```python
from build123d import *

# Parameters (mm, degrees)
SKETCH_2_W          = 66
SKETCH_2_H          = 32
EXTRUDE_1_DEPTH     = 5
SKETCH_3_W          = 46
SKETCH_3_H          = 11.5
CUT_EXTRUDE_2_DEPTH = 38.013511047
SKETCH_4_W          = 5
SKETCH_4_H          = 11.5
CUT_EXTRUDE_3_DEPTH = 69.095521145
SKETCH_5_W          = 10
SKETCH_5_H          = 32
EXTRUDE_2_DEPTH     = 5
SKETCH_6_W          = 10
SKETCH_6_H          = 32
EXTRUDE_3_DEPTH     = 3
SKETCH_7_R          = 1.5
CUT_EXTRUDE_4_DEPTH = 39.013155617
CHAMFER_1_SIZE      = 2
CHAMFER_2_SIZE      = 1


with BuildPart() as part:
    # Sketch 2 → Extrude 1 (new body)
    with BuildSketch(Plane(origin=(0, 0, 0), x_dir=(0, 0, -1), z_dir=(1, 0, 0))):
        Rectangle(SKETCH_2_W, SKETCH_2_H)
    extrude(amount=EXTRUDE_1_DEPTH)

    # Sketch 3 → Cut-Extrude 2 (cut, through all)
    with BuildSketch(Plane.ZY):
        Rectangle(SKETCH_3_W, SKETCH_3_H)
    extrude(amount=-CUT_EXTRUDE_2_DEPTH, mode=Mode.SUBTRACT)

    # Sketch 4 → Cut-Extrude 3 (cut, through all)
    with BuildSketch(Plane(origin=(0, 0, -33), x_dir=(-1, 0, 0), z_dir=(0, 0, -1))):
        with Locations((-2.5, 0)):
            Rectangle(SKETCH_4_W, SKETCH_4_H)
    extrude(amount=-CUT_EXTRUDE_3_DEPTH, mode=Mode.SUBTRACT)


with BuildPart() as cut_extrude_3_piece_1:
    # of the separate pieces the step leaves, piece 1, a body of its own (cut_extrude_3_pieces)
    add(part.part.solids().sort_by_distance((0, -16, -33))[0])



with BuildPart() as cut_extrude_3_piece_2:
    # of the separate pieces the step leaves, piece 2, a body of its own (cut_extrude_3_pieces)
    add(part.part.solids().sort_by_distance((0, 16, -33))[0])


with BuildPart() as cut_extrude_3_piece_1_1:
    add(cut_extrude_3_piece_1.part)

    add(cut_extrude_3_piece_2.part)  # Extrude 2 merges Cut-Extrude 3 piece 2
    # Sketch 5 → Extrude 2 (add)
    with BuildSketch(Plane(origin=(5, 0, 0), x_dir=(0, 0, -1), z_dir=(1, 0, 0))):
        with Locations((28, 0)):
            Rectangle(SKETCH_5_W, SKETCH_5_H)
    extrude(amount=EXTRUDE_2_DEPTH)

    # Sketch 6 → Extrude 3 (add)
    with BuildSketch(Plane(origin=(5, 0, 0), x_dir=(0, 0, -1), z_dir=(1, 0, 0))):
        with Locations((-28, 0)):
            Rectangle(SKETCH_6_W, SKETCH_6_H)
    extrude(amount=EXTRUDE_3_DEPTH)

    # Sketch 7 → Cut-Extrude 4 (cut, through all)
    with BuildSketch(Plane.ZY):
        with Locations((-16.25, 8.75)):
            Circle(SKETCH_7_R)
        with Locations((16.25, 8.75)):
            Circle(SKETCH_7_R)
        with Locations((16.25, -8.75)):
            Circle(SKETCH_7_R)
        with Locations((-16.25, -8.75)):
            Circle(SKETCH_7_R)
    extrude(amount=-CUT_EXTRUDE_4_DEPTH, mode=Mode.SUBTRACT)

    # Chamfer 1
    # the kernel refuses this chamfer: 2 mm, written as the material it takes off along each edge
    with BuildSketch(Plane(origin=(0, -8.75, -16.25), x_dir=(0, 0, 1), z_dir=(0, -1, 0))) as chamfer_1_piece_1:
        Polygon((1.5 + CHAMFER_1_SIZE, 0), (1.5, -CHAMFER_1_SIZE), (1.5, 0), align=None)
    revolve(axis=Axis((0, -8.75, -16.25), (-1, 0, 0)), mode=Mode.SUBTRACT)
    with BuildSketch(Plane(origin=(0, -8.75, 16.25), x_dir=(0, 0, 1), z_dir=(0, -1, 0))) as chamfer_1_piece_2:
        Polygon((1.5 + CHAMFER_1_SIZE, 0), (1.5, -CHAMFER_1_SIZE), (1.5, 0), align=None)
    revolve(axis=Axis((0, -8.75, 16.25), (-1, 0, 0)), mode=Mode.SUBTRACT)
    with BuildSketch(Plane(origin=(0, 8.75, 16.25), x_dir=(0, 0, 1), z_dir=(0, -1, 0))) as chamfer_1_piece_3:
        Polygon((1.5 + CHAMFER_1_SIZE, 0), (1.5, -CHAMFER_1_SIZE), (1.5, 0), align=None)
    revolve(axis=Axis((0, 8.75, 16.25), (-1, 0, 0)), mode=Mode.SUBTRACT)
    with BuildSketch(Plane(origin=(0, 8.75, -16.25), x_dir=(0, 0, 1), z_dir=(0, -1, 0))) as chamfer_1_piece_4:
        Polygon((1.5 + CHAMFER_1_SIZE, 0), (1.5, -CHAMFER_1_SIZE), (1.5, 0), align=None)
    revolve(axis=Axis((0, 8.75, -16.25), (-1, 0, 0)), mode=Mode.SUBTRACT)

    # Chamfer 2
    chamfer_2_edges = [cut_extrude_3_piece_1_1.edges().sort_by_distance(p)[0] for p in [
        (5, 16, -33),
        (10, -16, -28),
        (10, 0, -33),
        (10, 16, -28),
        (4, 16, 33),
        (5, -16, -33),
        (4, -16, 33),
        (8, 0, 33),
        (8, -16, 28),
        (8, 16, 28),
    ]]
    chamfer(chamfer_2_edges, length=CHAMFER_2_SIZE)


solid = cut_extrude_3_piece_1_1.part
```
Could you check a few things on this model? Use its own coordinates, in mm. A direction names the side the tool comes from. Round coordinates to 2 decimals unless told otherwise and drop trailing zeros. Write each loop counter-clockwise with the first axis right and the second up, starting at its lowest first coordinate (ties: lowest second). Pieces come first, ordered by that corner, then holes. Notation, with made-up numbers: M 8.25,69 L 17.25,69 A16 cw 17.25,93 Z; hole C 17.25,67.5 d4. An arc over 180 degrees is marked long. Write each question's results on one line, items separated by ' | '. Start each with the question number.
1. I need wall thicknesses on L1, parallel to Y at x = 4.1, z = -16.25; L2, parallel to Z at x = 5.25, y = 13.5; L3, parallel to Y at x = 4.75, z = -27. Which ranges of each line are inside material? Lowest first, please. Write a range as from..to.
2. I'm going to push flat-ended pins straight in: pin 1 Ø8 at (y, z) = (10.5, 9) entering from +X; pin 2 Ø5 at (x, y) = (4, 5.5) entering from +Z; pin 3 Ø5 at (y, z) = (8.75, -16.25) entering from -X; pin 4 Ø7 at (y, z) = (-3.5, 27) entering from +X. Where does each tip first touch, or does it pass through?
3. Imagine slicing it at C-C on y = -8.75. List the corners of the cut face in (x, z) for me, and give its area (3 significant figures).
4. Imagine slicing it at A-A on y = -2. List the corners of the cut face in (x, z) for me.
5. Imagine slicing it at D-D on z = -4. List the corners of the cut face in (x, y) for me.
6. Imagine slicing it at B-B on z = -16.25. List the corners of the cut face in (x, y) for me.
7. On a 3-axis mill with a long thin cutter (end or side, diameter ignored), from which of +Z, -Z, +X, -X, +Y, -Y can I reach the whole of each face in a straight line? I mean faces 5 (the face through (3, -5.75, 0)), 6 (the face through (8, 0, 28)), 7 (the face through (6, 0, 23)). Say none if no direction works.
8. Thinking about a two-plate mould opening in Y: for faces 1 (the face through (3.48, 8.82, -17.75)), 2 (the face through (3.48, -9.66, 15.06)), 3 (the face through (5, -11, 0)), 4 (the face through (2, 16, 0)), which applies, +Y half, -Y half, draft (parallel to the pull), parting line (faces both ways), or undercut?
Result sheet:
1) L1: y = -16..-10.25, -7.25..-5.75, 5.75..7.25, 10.25..16 | L2: z = -33..-23, 23..33 | L3: y = -16..-5.75, 5.75..16
2) pin 1: stops at x = 5 | pin 2: stops at z = 33 | pin 3: stops at x = 1 | pin 4: stops at x = 8
3) outline: M 0,-33 L 9,-33 L 10,-32 L 10,-23 L 5,-23 L 5,-17.75 L 2,-17.75 L 0,-19.75 Z; M 0,-12.75 L 2,-14.75 L 5,-14.75 L 5,14.75 L 2,14.75 L 0,12.75 Z; M 0,19.75 L 2,17.75 L 5,17.75 L 5,23 L 8,23 L 8,32 L 7,33 L 0,33 Z | area: 371 mm^2
4) outline: M 5,-33 L 9,-33 L 10,-32 L 10,-23 L 5,-23 Z; M 5,23 L 8,23 L 8,32 L 7,33 L 5,33 Z
5) outline: M 0,-16 L 5,-16 L 5,-5.75 L 0,-5.75 Z; M 0,5.75 L 5,5.75 L 5,16 L 0,16 Z
6) outline: M 0,-16 L 5,-16 L 5,-10.25 L 2,-10.25 L 0,-12.25 Z; M 0,12.25 L 2,10.25 L 5,10.25 L 5,16 L 0,16 Z; M 0.5,-5.75 L 2,-7.25 L 5,-7.25 L 5,-5.75 Z; M 0.5,5.75 L 5,5.75 L 5,7.25 L 2,7.25 Z
7) face 5: +Z, -Z, -X | face 6: +Z, +X, +Y, -Y | face 7: +X, +Y, -Y
8) face 1: undercut | face 2: undercut | face 3: draft | face 4: +Y half
